from build123d import *

# Parameters (mm, degrees)
F1_DEPTH = 12.7
F2_DEPTH = 63.5
F3_DEPTH = 25.4
F5_R     = 6.35


with BuildPart() as f1:
    # F0 (on Front) → F1 (new body, symmetric)
    with BuildSketch(Plane.XZ):
        with BuildLine():
            add(Edge.make_bspline(
                [(-41.275, 9.525), (-35.564307, 57.795133), (-13.679589, 63.100524), (47.681865, 61.9252)],
                knots=[0, 0, 0, 0, 103.242941, 103.242941, 103.242941, 103.242941], degree=3))
            Line((-41.275, 9.525), (22.225, 9.525))
            Line((22.225, 9.525), (22.225, 36.468335))
            ThreePointArc((22.225, 36.468335), (29.681143, 54.469057), (47.681865, 61.9252))
        make_face()
        Polygon((22.225, 9.525), (-41.275, 9.525), (-41.275, -9.525), (41.275, -9.525), (41.275, 9.525), align=None)
        with BuildLine():
            Line((22.225, 36.468335), (22.225, 9.525))
            Line((22.225, 9.525), (41.275, 9.525))
            Line((41.275, 9.525), (41.275, 36.468335))
            ThreePointArc((41.275, 36.468335), (43.151527, 40.998673), (47.681865, 42.8752))
            Line((47.681865, 42.8752), (66.902457, 42.8752))
            Line((66.902457, 42.8752), (66.902457, 61.9252))
            Line((66.902457, 61.9252), (47.681865, 61.9252))
            ThreePointArc((47.681865, 61.9252), (29.681143, 54.469057), (22.225, 36.468335))
        make_face()
        Polygon((66.902457, 66.675), (66.902457, 61.9252), (66.902457, 42.8752), (66.902457, 38.090521), (117.702457, 38.090521), (117.702457, 66.675), align=None)
    extrude(amount=F1_DEPTH, both=True)

    # F0 (on Front) → F2 (join, symmetric)
    with BuildSketch(Plane.XZ):
        Polygon((22.225, 9.525), (-41.275, 9.525), (-41.275, -9.525), (41.275, -9.525), (41.275, 9.525), align=None)
    extrude(amount=F2_DEPTH, both=True)

    # F0 (on Front) → F3 (join)
    with BuildSketch(Plane.XZ):
        with BuildLine():
            add(Edge.make_bspline(
                [(-41.275, 9.525), (-35.564307, 57.795133), (-13.679589, 63.100524), (47.681865, 61.9252)],
                knots=[0, 0, 0, 0, 103.242941, 103.242941, 103.242941, 103.242941], degree=3))
            Line((-41.275, 9.525), (22.225, 9.525))
            Line((22.225, 9.525), (22.225, 36.468335))
            ThreePointArc((22.225, 36.468335), (29.681143, 54.469057), (47.681865, 61.9252))
        make_face()
        Polygon((22.225, 9.525), (-41.275, 9.525), (-41.275, -9.525), (41.275, -9.525), (41.275, 9.525), align=None)
        with BuildLine():
            Line((22.225, 36.468335), (22.225, 9.525))
            Line((22.225, 9.525), (41.275, 9.525))
            Line((41.275, 9.525), (41.275, 36.468335))
            ThreePointArc((41.275, 36.468335), (43.151527, 40.998673), (47.681865, 42.8752))
            Line((47.681865, 42.8752), (66.902457, 42.8752))
            Line((66.902457, 42.8752), (66.902457, 61.9252))
            Line((66.902457, 61.9252), (47.681865, 61.9252))
            ThreePointArc((47.681865, 61.9252), (29.681143, 54.469057), (22.225, 36.468335))
        make_face()
        Polygon((66.902457, 66.675), (66.902457, 61.9252), (66.902457, 42.8752), (66.902457, 38.090521), (117.702457, 38.090521), (117.702457, 66.675), align=None)
    extrude(amount=F3_DEPTH)

    # F0 (on Front) → F4 (revolve)
    with BuildSketch(Plane.XZ):
        Polygon((66.902457, 66.675), (66.902457, 61.9252), (66.902457, 42.8752), (66.902457, 38.090521), (117.702457, 38.090521), (117.702457, 66.675), align=None)
    revolve(axis=Axis((117.702457, 0, 52.382761), (0, 0, 1)))

    # F5
    f5_edges = [f1.edges().sort_by_distance(p)[0] for p in [
        (-41.275, -63.5, 0),
        (41.275, -63.5, 0),
        (-41.275, 63.5, 0),
        (41.275, 63.5, 0),
    ]]
    fillet(f5_edges, radius=F5_R)


solid = f1.part
Work out the finished part from the listing and answer in its coordinate system (mm). A direction names the side the tool comes from. Coordinates: 2 decimals unless noted, no trailing zeros. Loops run counter-clockwise (first coordinate to the right, second up) from the corner with the lowest first, then second, coordinate; pieces in that order, holes last. Notation, with made-up numbers: (19.25, -6.75) -> (47.25, -6.75) arc R18 cw to (47.25, 21.25) -> close; hole circle Ø8 at (-6, 56.5). An arc over 180 degrees is marked (long way). Answer as CSV lines item,"result".
1) The part is cut by section B-B (z = -2). Give the vertices of the cut face in (x, y) (3 decimals).
A:
outline,"(-41.275, -57.15) arc R6.35 ccw to (-34.925, -63.5) -> (34.925, -63.5) arc R6.35 ccw to (41.275, -57.15) -> (41.275, 57.15) arc R6.35 ccw to (34.925, 63.5) -> (-34.925, 63.5) arc R6.35 ccw to (-41.275, 57.15) -> close"
2) For a pull along X with two mould halves and no side action, classify faces 1 (the face through (66.902, -6, 41)), 2 (the face through (39.365, 61.689, 0.133)), 3 (the face through (168.264, 4.915, 52.183)) as released by +X, released by -X, zero draft, split by the parting line, or undercut.
A:
face 1,"undercut"
face 2,"released by +X"
face 3,"split by the parting line"
3) The part is cut by section D-D (x = 129). Give the vertices of the cut face in (y, z) (3 decimals), and give its area (3 significant figures).
A:
outline,"(-49.528, 38.091) -> (49.528, 38.091) -> (49.528, 66.675) -> (-49.528, 66.675) -> close"
area,"2,830 mm²"
4) The part is cut by section A-A (y = 40). Give the vertices of the cut face in (x, z) (3 decimals).
A:
outline,"(-41.275, -9.525) -> (41.275, -9.525) -> (41.275, 9.525) -> (-41.275, 9.525) -> close; (86.387, 38.091) -> (149.018, 38.091) -> (149.018, 66.675) -> (86.387, 66.675) -> close"
5) The part is cut by section C-C (y = -45). Give the vertices of the cut face in (x, z) (3 decimals), and give its area (3 significant figures).
A:
outline,"(-41.275, -9.525) -> (41.275, -9.525) -> (41.275, 9.525) -> (-41.275, 9.525) -> close; (94.13, 38.091) -> (141.274, 38.091) -> (141.274, 66.675) -> (94.13, 66.675) -> close"
area,"2,920 mm²"
6) Flat-ended cylindrical pins translate along their axes: pin 1 (6 mm diameter, centred on y = 41, z = 44.5, fed in from -X); pin 2 (14 mm diameter, centred on y = 13, z = 10.5, fed in from +X) (3 decimals); pin 3 (21 mm diameter, centred on x = 55, y = 2, fed in from -Z); pin 4 (10 mm diameter, centred on y = 32.5, z = 11.5, fed in from -X) (3 decimals). Find the tip coordinate at first contact, or state that the pin passes through.
A:
pin 1,"stops at x = 83.99"
pin 2,"stops at x = 41.275"
pin 3,"stops at z = 42.03"
pin 4,"stops at x = -41.275"
7) For faces 4 (the face through (14, 12.7, 32)), 5 (the face through (41.275, -1, 8)), 6 (the face through (1, 38, 9.525)), determine the directions among +Z, -Z, +X, -X, +Y, -Y from which every point of the face is accessible in a straight line to the end or side of a thin tool.
A:
face 4,"+Z, -X, +Y"
face 5,"-Z, +X, +Y, -Y"
face 6,"+Z, +X, -X, +Y"
8) Straight lines are drawn through the part: probe 1 along X at (y, z) = (-24.5, 4) (3 decimals); probe 2 along Y at (x, z) = (-30, 17.5); probe 3 along Z at (x, y) = (-20, -48) (3 decimals). For each, find the intervals that lie inside material, in ascending order.
A:
probe 1,"x = -41.275 to 41.275"
probe 2,"y = -25.4 to 12.7"
probe 3,"z = -9.525 to 9.525"
